```python
from build123d import *

# Parameters (mm, degrees)
SKETCH1_W           = 44.5
SKETCH1_H           = 134.5
BOSS_EXTRUDE1_DEPTH = 18
BOSS_EXTRUDE2_DEPTH = 7
SKETCH5_R           = 2.5
BOSS_EXTRUDE4_DEPTH = 25


with BuildPart() as part:
    # Sketch1 → Boss-Extrude1 (new body)
    with BuildSketch(Plane(origin=(0, 0, 0), x_dir=(1, 0, 0), z_dir=(0, 1, 0))):
        Rectangle(SKETCH1_W, SKETCH1_H)
    extrude(amount=BOSS_EXTRUDE1_DEPTH)

    # Sketch3 → Boss-Extrude2 (add)
    with BuildSketch(Plane.XY.offset(67.25)):
        with BuildLine():
            Line((-22.25, 14.488612788), (-22.25, 3.511387212))
            ThreePointArc((-22.25, 3.511387212), (-24.031009601, 4.395950378), (-24.75, 6.25))
            Line((-24.75, 6.25), (-24.75, 11.75))
            ThreePointArc((-24.75, 11.75), (-24.031009601, 13.604049622), (-22.25, 14.488612788))
        make_face()
    extrude(amount=-BOSS_EXTRUDE2_DEPTH)

    # Sketch5 → Boss-Extrude4 (add)
    with BuildSketch(Plane.XY.offset(67.25)):
        with Locations(Location((-22, 11.75, 0), (0, 0, 180))):
            Circle(SKETCH5_R)
        with Locations(Location((-22, 6.25, 0), (0, 0, 180))):
            Circle(SKETCH5_R)
    extrude(amount=BOSS_EXTRUDE4_DEPTH)


solid = part.part
```
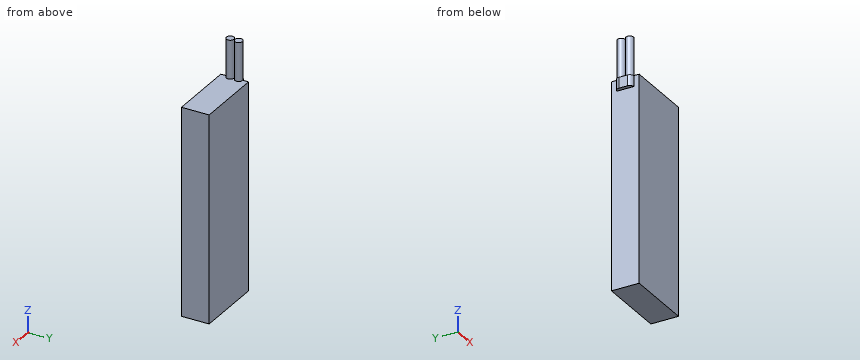
Verification items for the finished model (mm, model axes). Give positions to 0.01 mm unless a question says otherwise; leave off trailing zeros. Order: outer loops, then holes, each group sorted by start corner. A loop starts at its lowest first (then second) coordinate and runs counter-clockwise, first axis right, second up. Notation, with made-up numbers: (-24, 63) - (12, 63) arc R21 cw to (12, 88) - close; hole circle Ø9 at (0.25, 60.25). An arc over 180 degrees is marked (long way). Answer as CSV lines item,"result". Start each with the question number.
Item 1: Material ranges on L1, parallel to X at y = 9, z = 28; L2, parallel to Z at x = 3.5, y = 6.75; L3, parallel to X at y = 9.75, z = 77.5, recorded low to high.
Item 2: Section check B-B, the plane y = 2. Record the boundary of the cut face in (x, z).
Item 3: Section check A-A, the plane z = -44. Record the boundary of the cut face in (x, y).
Item 4: Gauge pin test, flat ends, axial feed: pin 1 (3 mm diameter, centred on y = 15.5, z = 3.5, fed in from -X); pin 2 (5 mm diameter, centred on y = 4, z = 75, fed in from -X); pin 3 (0.8 mm diameter, centred on x = -23.5, y = 9, fed in from -Z). Record the tip position at first contact, or that the pin passes through.
Filled in:
1,L1,"-22.25 to 22.25"
1,L2,"-67.25 to 67.25"
1,L3,"-23.5 to -20.5"
2,outline,"(-22.25, -67.25) - (22.25, -67.25) - (22.25, 67.25) - (-22.25, 67.25) - close"
3,outline,"(-22.25, 0) - (22.25, 0) - (22.25, 18) - (-22.25, 18) - close"
4,pin 1,"x = -22.25"
4,pin 2,"x = -24.5"
4,pin 3,"z = 60.25"
